from build123d import *

# Parameters (mm, degrees)
SKETCH1_W                 = 29
SKETCH1_H                 = 27
BOSS_EXTRUDE2_DEPTH       = 2
SKETCH2_W                 = 2
SKETCH2_H                 = 27
BOSS_EXTRUDE3_DEPTH       = 27
SKETCH3_W                 = 2
SKETCH3_H                 = 27
BOSS_EXTRUDE4_DEPTH       = 27
SKETCH4_W                 = 2
SKETCH4_H                 = 27
BOSS_EXTRUDE5_DEPTH       = 29
SKETCH5_W                 = 29
SKETCH5_H                 = 2
BOSS_EXTRUDE6_DEPTH       = 5
SKETCH6_W                 = 29
SKETCH6_H                 = 2
BOSS_EXTRUDE7_DEPTH       = 5
SKETCH7_W                 = 29
SKETCH7_H                 = 2
BOSS_EXTRUDE9_DEPTH       = 3
SKETCH8_W                 = 29
SKETCH8_H                 = 70
BOSS_EXTRUDE10_DEPTH      = 3
SKETCH9_W                 = 29
SKETCH9_H                 = 70
BOSS_EXTRUDE11_DEPTH      = 3
SKETCH10_R                = 1.75
CUT_EXTRUDE1_DEPTH        = 40
CUT_EXTRUDE1_DEPTH_BACK   = 4
SKETCH14_W                = 64.059186105
SKETCH14_H                = 2.228166541
BOSS_EXTRUDE15_DEPTH      = 50
SKETCH15_W                = 64.059186105
SKETCH15_H                = 2.228166541
BOSS_EXTRUDE16_DEPTH      = 50
SKETCH16_W                = 17.5
SKETCH16_H                = 2.228166541
BOSS_EXTRUDE17_DEPTH      = 29
BOSS_EXTRUDE18_DEPTH      = 1
BOSS_EXTRUDE18_DEPTH_BACK = 1
SKETCH19_W                = 29
SKETCH19_H                = 43
CUT_EXTRUDE2_DEPTH        = 15
SKETCH20_W                = 10
SKETCH20_H                = 64.059186105
BOSS_EXTRUDE19_DEPTH      = 3
SKETCH21_R                = 1.75
BOSS_EXTRUDE20_DEPTH      = 4


with BuildPart() as part:
    # Sketch1 → Boss-Extrude2 (new body)
    with BuildSketch(Plane.XY):
        with Locations((14.5, 13.5)):
            Rectangle(SKETCH1_W, SKETCH1_H)
    extrude(amount=BOSS_EXTRUDE2_DEPTH)

    # Sketch2 → Boss-Extrude3 (add)
    with BuildSketch(Plane.XY):
        with Locations((1, 13.5)):
            Rectangle(SKETCH2_W, SKETCH2_H)
    extrude(amount=-BOSS_EXTRUDE3_DEPTH)

    # Sketch3 → Boss-Extrude4 (add)
    with BuildSketch(Plane.XY):
        with Locations((28, 13.5)):
            Rectangle(SKETCH3_W, SKETCH3_H)
    extrude(amount=-BOSS_EXTRUDE4_DEPTH)

    # Sketch4 → Boss-Extrude5 (add)
    with BuildSketch(Plane(origin=(0, 0, 0), x_dir=(0, 0, -1), z_dir=(1, 0, 0))):
        with Locations((26, 13.5)):
            Rectangle(SKETCH4_W, SKETCH4_H)
    extrude(amount=BOSS_EXTRUDE5_DEPTH)

    # Sketch5 → Boss-Extrude6 (add)
    with BuildSketch(Plane(origin=(0, 0, 0), x_dir=(0, 0, -1), z_dir=(1, 0, 0))):
        with Locations((12.5, 26)):
            Rectangle(SKETCH5_W, SKETCH5_H)
    extrude(amount=BOSS_EXTRUDE6_DEPTH)

    # Sketch6 → Boss-Extrude7 (add)
    with BuildSketch(Plane(origin=(29, 0, 0), x_dir=(0, 0, -1), z_dir=(1, 0, 0))):
        with Locations((12.5, 26)):
            Rectangle(SKETCH6_W, SKETCH6_H)
    extrude(amount=-BOSS_EXTRUDE7_DEPTH)

    # Sketch7 → Boss-Extrude9 (add)
    with BuildSketch(Plane.XY):
        with Locations((14.5, 26)):
            Rectangle(SKETCH7_W, SKETCH7_H)
    extrude(amount=-BOSS_EXTRUDE9_DEPTH)

    # Sketch8 → Boss-Extrude10 (add)
    with BuildSketch(Plane(origin=(0, 0, 0), x_dir=(0, 0, -1), z_dir=(1, 0, 0))):
        with Locations((12.5, 35)):
            Rectangle(SKETCH8_W, SKETCH8_H)
    extrude(amount=-BOSS_EXTRUDE10_DEPTH)

    # Sketch9 → Boss-Extrude11 (add)
    with BuildSketch(Plane(origin=(29, 0, 0), x_dir=(0, 0, -1), z_dir=(1, 0, 0))):
        with Locations((12.5, 35)):
            Rectangle(SKETCH9_W, SKETCH9_H)
    extrude(amount=BOSS_EXTRUDE11_DEPTH)

    # Sketch10 → Cut-Extrude1 (cut, two sides)
    with BuildSketch(Plane(origin=(0, 0, 0), x_dir=(0, 0, -1), z_dir=(1, 0, 0))) as cut_extrude1_sk:
        with Locations((12.5, 60)):
            Circle(SKETCH10_R)
    extrude(amount=CUT_EXTRUDE1_DEPTH, mode=Mode.SUBTRACT)
    extrude(cut_extrude1_sk.sketch, amount=-CUT_EXTRUDE1_DEPTH_BACK, mode=Mode.SUBTRACT)

    # Sketch14 → Boss-Extrude15 (add)
    with BuildSketch(Plane(origin=(29, 0, 0), x_dir=(0, 0, -1), z_dir=(1, 0, 0))):
        with Locations((12.529593053, 1.114083271)):
            Rectangle(SKETCH14_W, SKETCH14_H)
    extrude(amount=BOSS_EXTRUDE15_DEPTH)

    # Sketch15 → Boss-Extrude16 (add)
    with BuildSketch(Plane(origin=(0, 0, 0), x_dir=(0, 0, -1), z_dir=(1, 0, 0))):
        with Locations((12.529593053, 1.114083271)):
            Rectangle(SKETCH15_W, SKETCH15_H)
    extrude(amount=-BOSS_EXTRUDE16_DEPTH)

    # Sketch16 → Boss-Extrude17 (add)
    with BuildSketch(Plane(origin=(0, 0, 0), x_dir=(0, 0, -1), z_dir=(1, 0, 0))):
        with Locations((-10.75, 1.114083271)):
            Rectangle(SKETCH16_W, SKETCH16_H)
    extrude(amount=BOSS_EXTRUDE17_DEPTH)

    # Sketch18 → Boss-Extrude18 (add, two sides)
    with BuildSketch(Plane.XY.offset(-11)) as boss_extrude18_sk:
        Polygon((-35.241827575, 2.228166541), (-3, 2.228166541), (-3, 36.114083271), align=None)
        Polygon((32, 2.228166541), (65.471342827, 2.228166541), (32, 36.114083271), align=None)
    extrude(amount=BOSS_EXTRUDE18_DEPTH)
    extrude(boss_extrude18_sk.sketch, amount=-BOSS_EXTRUDE18_DEPTH_BACK)

    # Sketch19 → Cut-Extrude2 (cut)
    with BuildSketch(Plane(origin=(29, 0, 0), x_dir=(0, 0, -1), z_dir=(1, 0, 0))):
        with Locations((12.5, 48.5)):
            Rectangle(SKETCH19_W, SKETCH19_H)
    extrude(amount=CUT_EXTRUDE2_DEPTH, mode=Mode.SUBTRACT)

    # Sketch20 → Boss-Extrude19 (add)
    with BuildSketch(Plane(origin=(0, 0, 0), x_dir=(1, 0, 0), z_dir=(0, 1, 0))):
        with Locations((-41, 12.529593053)):
            Rectangle(SKETCH20_W, SKETCH20_H)
        with Locations((-27, 12.529593053)):
            Rectangle(SKETCH20_W, SKETCH20_H)
        with Locations((70, 12.529593053)):
            Rectangle(SKETCH20_W, SKETCH20_H)
        with Locations((56, 12.529593053)):
            Rectangle(SKETCH20_W, SKETCH20_H)
    extrude(amount=-BOSS_EXTRUDE19_DEPTH)

    # Sketch21 → Boss-Extrude20 (add)
    with BuildSketch(Plane(origin=(0, 0, 0), x_dir=(1, 0, 0), z_dir=(0, 1, 0))):
        with Locations((-41, 29.559186105)):
            Circle(SKETCH21_R)
        with Locations((-41, 12.559186105)):
            Circle(SKETCH21_R)
        with Locations((-41, -4.5)):
            Circle(SKETCH21_R)
        with Locations((-27, 29.559186105)):
            Circle(SKETCH21_R)
        with Locations((-27, 12.559186105)):
            Circle(SKETCH21_R)
        with Locations((-27, -4.5)):
            Circle(SKETCH21_R)
        with Locations((56, 29.559186105)):
            Circle(SKETCH21_R)
        with Locations((56, 12.559186105)):
            Circle(SKETCH21_R)
        with Locations((56, -4.5)):
            Circle(SKETCH21_R)
        with Locations((70, 29.559186105)):
            Circle(SKETCH21_R)
        with Locations((70, 12.559186105)):
            Circle(SKETCH21_R)
        with Locations((70, -4.5)):
            Circle(SKETCH21_R)
    extrude(amount=-BOSS_EXTRUDE20_DEPTH)


solid = part.part
Can you work these out from the model? Positions are in its coordinate system, mm. A direction names the side the tool comes from. Give positions to 0.01 mm unless a question says otherwise; leave off trailing zeros. Loops run counter-clockwise (first coordinate to the right, second up) from the corner with the lowest first, then second, coordinate; pieces in that order, holes last. Notation, with made-up numbers: (72, 69) -> (128, 69) arc R20 ccw to (128, 86) -> close; hole circle Ø6 at (54.5, 32.25). An arc over 180 degrees is marked (long way). Return JSON: item names as keys, results as strings.
Q1. We'd pull the mould along Z, two halves only. Please class faces 1 (the face through (77, 0, -12)), 2 (the face through (-12, 12, -10)), 3 (the face through (-28.29, -3.49, -30.74)): released by +Z, released by -Z, zero draft, split by the parting line, or undercut.
Checks:
{"face 1": "zero draft", "face 2": "released by +Z", "face 3": "undercut"}
Q2. I want a section at D-D, the plane z = 9. List the corners of the cut face in (x, y) for me, then the cut area to 3 significant figures.
Checks:
{"outline": "(-50, 0) -> (-46, 0) -> (-46, -3) -> (-36, -3) -> (-36, 0) -> (-32, 0) -> (-32, -3) -> (-22, -3) -> (-22, 0) -> (51, 0) -> (51, -3) -> (61, -3) -> (61, 0) -> (65, 0) -> (65, -3) -> (75, -3) -> (75, 0) -> (79, 0) -> (79, 2.23) -> (-50, 2.23) -> close", "area": "407 mm2"}
Q3. I want a section at C-C, the plane y = 60. List the corners of the cut face in (x, z) for me, then the cut area to 3 significant figures.
Checks:
{"outline": "(-3, -27) -> (0, -27) -> (0, -14.25) -> (-3, -14.25) -> close; (-3, -10.75) -> (0, -10.75) -> (0, 2) -> (-3, 2) -> close", "area": "76.5 mm2"}
Q4. For pin 1 Ø1.5 at (x, z) = (10.5, -26.5) entering from -Y; pin 2 Ø10 at (y, z) = (17, -13.5) entering from +X; pin 3 Ø6 at (y, z) = (15, -23) entering from -X, each with a flat end and sliding along its axis, tell me the tip position at first contact or that it passes through.
Checks:
{"pin 1": "stops at y = 0", "pin 2": "stops at x = 55.59", "pin 3": "stops at x = -3"}
Q5. On a 3-axis mill with a long thin cutter (end or side, diameter ignored), from which of +Z, -Z, +X, -X, +Y, -Y can I reach the whole of each face in a straight line? I mean faces 4 (the face through (0, 49, -12)), 5 (the face through (70, -4, 4)), 6 (the face through (14, 25, -2)), 7 (the face through (51, -1, -12)), 8 (the face through (-3, 37, -12)). Say none if no direction works.
Checks:
{"face 4": "+Z, -Z, +X, +Y", "face 5": "+Z, -Z, +X, -X, -Y", "face 6": "-Y", "face 7": "+Z, -Z, -Y", "face 8": "-X, +Y"}
Q6. I need wall thicknesses on probe 1 along X at (y, z) = (-1, 0); probe 2 along Y at (x, z) = (32, 2); probe 3 along X at (y, z) = (41.5, -9). Which ranges of each line are inside material? Lowest first, please.
Checks:
{"probe 1": "x = -46 to -36, -32 to -22, 51 to 61, 65 to 75", "probe 2": "y = 0 to 2.23", "probe 3": "x = -3 to 0"}
Q7. I want a section at B-B, the plane x = 8. List the corners of the cut face in (y, z) for me, then the cut area to 3 significant figures.
Checks:
{"outline": "(0, -27) -> (27, -27) -> (27, -25) -> (0, -25) -> close; (0, 0) -> (25, 0) -> (25, -3) -> (27, -3) -> (27, 2) -> (2.23, 2) -> (2.23, 19.5) -> (0, 19.5) -> close", "area": "153 mm2"}
